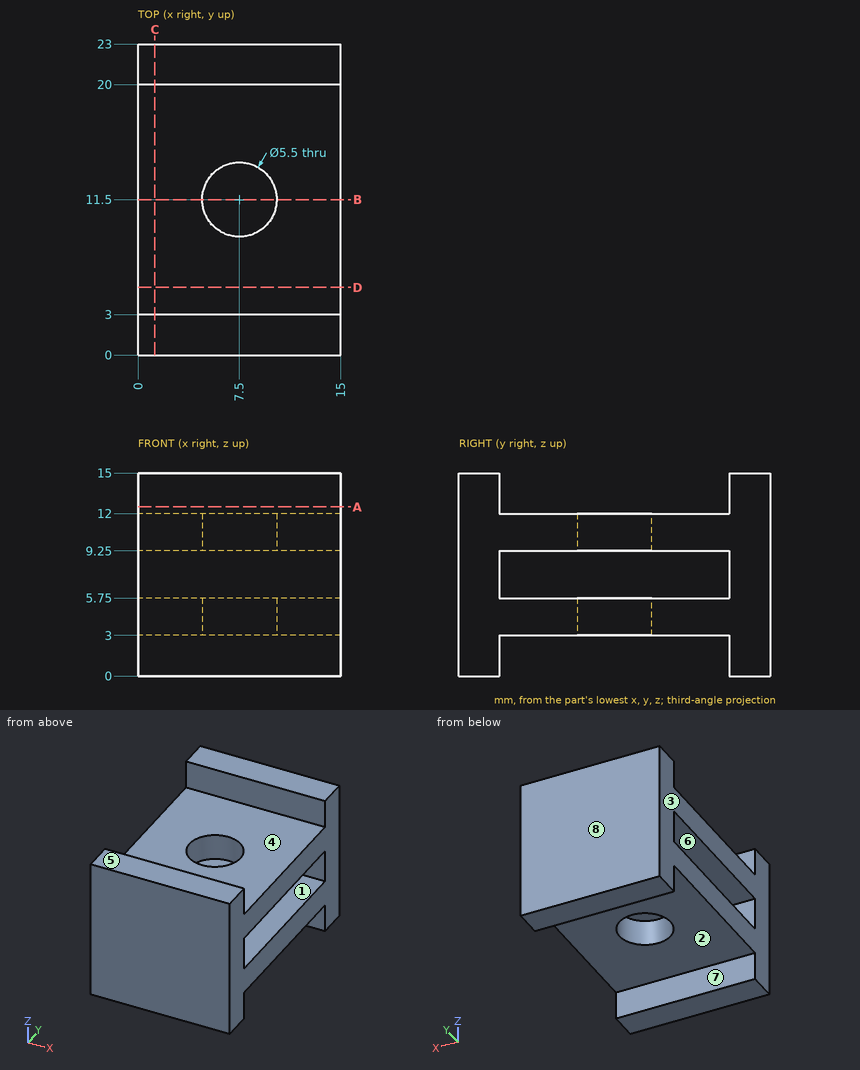
Geometry check sheet. Reference: drawing and pictorial views, mm from the part's lowest x, y, z. A direction names the side the tool comes from. Give positions to 0.01 mm unless a question says otherwise; leave off trailing zeros. Order: outer loops, then holes, each group sorted by start corner. A loop starts at its lowest first (then second) coordinate and runs counter-clockwise, first axis right, second up. Notation, with made-up numbers: (25.25, 39) -> (52.25, 39) arc R27 ccw to (52.25, 72) -> close; hole circle Ø2 at (49.5, -32). An arc over 180 degrees is marked (long way). Use CSV: the item, a comma, the result in double quotes. Start each with the question number.
1) Sectioned sample at C-C, the plane x = 1.25. Record the boundary of the cut face in (y, z).
2) Sectioned sample at B-B, the plane y = 11.5. Record the boundary of the cut face in (x, z).
3) Set-up check for the marked faces 4, 5, 6, 7 and 8: record each of +Z, -Z, +X, -X, +Y, -Y from which the full face is reachable in a straight line by a thin tool's end or side.
4) Go/stop test with flat-tipped pins: P1, Ø1.5, axis at x = 8, z = 2, coming from the -Y side; P2, Ø6.5, axis at x = 7.5, y = 11.5, coming from the +Z side; P3, Ø7.5, axis at x = 8, y = 10, coming from the -Z side. Record where each tip stops, or that it passes through.
5) Mould release check, pull along Z, two halves, no side actions. Record for the marked faces 1, 2 and 3: released by +Z, released by -Z, zero draft, split by the parting line, or undercut.
6) Sectioned sample at D-D, the plane y = 5. Record the boundary of the cut face in (x, z), plus the area to 3 significant figures.
7) Sectioned sample at A-A, the plane z = 12.5. Record the boundary of the cut face in (x, y).
8) Material ranges on line 1 (Z direction, x = 9.25, y = 18.75); line 2 (X direction, y = 11.5, z = 5.15); line 3 (Y direction, x = 3, z = 14), recorded low to high. Write a range as from..to.
Recorded:
1,outline,"(0, 0) -> (3, 0) -> (3, 3) -> (20, 3) -> (20, 0) -> (23, 0) -> (23, 15) -> (20, 15) -> (20, 12) -> (3, 12) -> (3, 15) -> (0, 15) -> close; hole (3, 5.75) -> (20, 5.75) -> (20, 9.25) -> (3, 9.25) -> close"
2,outline,"(0, 3) -> (4.75, 3) -> (4.75, 5.75) -> (0, 5.75) -> close; (0, 9.25) -> (4.75, 9.25) -> (4.75, 12) -> (0, 12) -> close; (10.25, 3) -> (15, 3) -> (15, 5.75) -> (10.25, 5.75) -> close; (10.25, 9.25) -> (15, 9.25) -> (15, 12) -> (10.25, 12) -> close"
3,face 4,"+Z, +X, -X"
3,face 5,"+Z, +X, -X, +Y, -Y"
3,face 6,"+X, -X"
3,face 7,"-Z, +X, -X"
3,face 8,"+Z, -Z, +X, -X, +Y"
4,P1,"y = 0"
4,P2,"z = 12"
4,P3,"z = 3"
5,face 1,"undercut"
5,face 2,"released by -Z"
5,face 3,"zero draft"
6,outline,"(0, 3) -> (15, 3) -> (15, 5.75) -> (0, 5.75) -> close; (0, 9.25) -> (15, 9.25) -> (15, 12) -> (0, 12) -> close"
6,area,"82.5 mm2"
7,outline,"(0, 0) -> (15, 0) -> (15, 3) -> (0, 3) -> close; (0, 20) -> (15, 20) -> (15, 23) -> (0, 23) -> close"
8,line 1,"3..5.75, 9.25..12"
8,line 2,"0..4.75, 10.25..15"
8,line 3,"0..3, 20..23"
